Input: part model. Units: mm. Frame: model coordinates. A direction names the side the tool comes from. Give positions to 0.01 mm unless a question says otherwise; leave off trailing zeros. Write each loop counter-clockwise with the first axis right and the second up, starting at its lowest first coordinate (ties: lowest second). Pieces come first, ordered by that corner, then holes.
```python
from build123d import *

# Parameters (mm, degrees)
SKETCH21_R              = 5
CUT_EXTRUDE3_DEPTH      = 210.892061542
CUT_EXTRUDE3_DEPTH_BACK = 10.5


with BuildPart() as part:
    # Sweep-Thin3: sweep along a curve in space
    with BuildLine() as sweep_thin3_path:
        Line((0, 0, 0), (150, 0, 0))
        Line((150, 0, 0), (335.07515147, 200, 500))
        Line((335.07515147, 200, 500), (335.07515147, 200, 530))
    # Sketch2 → Sweep-Thin3 (sweep)
    with BuildSketch(Plane(origin=(0, 0, 0), x_dir=(0, 0, -1), z_dir=(1, 0, 0))):
        with BuildLine():
            Line((1.5, 9.5), (-1.5, 9.5))
            ThreePointArc((-1.5, 9.5), (-7.156854249, 7.156854249), (-9.5, 1.5))
            Line((-9.5, 1.5), (-9.5, -1.5))
            ThreePointArc((-9.5, -1.5), (-7.156854249, -7.156854249), (-1.5, -9.5))
            Line((-1.5, -9.5), (1.5, -9.5))
            ThreePointArc((1.5, -9.5), (7.156854249, -7.156854249), (9.5, -1.5))
            Line((9.5, -1.5), (9.5, 1.5))
            ThreePointArc((9.5, 1.5), (7.156854249, 7.156854249), (1.5, 9.5))
        make_face()
        with BuildLine():
            Line((1.5, 6.5), (-1.5, 6.5))
            ThreePointArc((-1.5, 6.5), (-5.035533906, 5.035533906), (-6.5, 1.5))
            Line((-6.5, 1.5), (-6.5, -1.5))
            ThreePointArc((-6.5, -1.5), (-5.035533906, -5.035533906), (-1.5, -6.5))
            Line((-1.5, -6.5), (1.5, -6.5))
            ThreePointArc((1.5, -6.5), (5.035533906, -5.035533906), (6.5, -1.5))
            Line((6.5, -1.5), (6.5, 1.5))
            ThreePointArc((6.5, 1.5), (5.035533906, 5.035533906), (1.5, 6.5))
        make_face(mode=Mode.SUBTRACT)
    sweep(path=sweep_thin3_path.line, transition=Transition.RIGHT)

    # Sketch21 → Cut-Extrude3 (cut, two sides)
    with BuildSketch(Plane(origin=(0, 0, 0), x_dir=(1, 0, 0), z_dir=(0, 1, 0))) as cut_extrude3_sk:
        with Locations((50, 0)):
            Circle(SKETCH21_R)
    extrude(amount=CUT_EXTRUDE3_DEPTH, mode=Mode.SUBTRACT)
    extrude(cut_extrude3_sk.sketch, amount=-CUT_EXTRUDE3_DEPTH_BACK, mode=Mode.SUBTRACT)


solid = part.part
```
Q1. Material intervals for line 1 along X through (y, z) = (-7, 0); line 2 along X through (y, z) = (-8.35, 0); line 3 along Z through (x, y) = (50, 7), sorted ascending.
Q2. Pin query (flat end, axial travel): pin 1 (0.9 mm diameter, centred on x = 26.5, z = -0.5, fed in from +Y); pin 2 (1.5 mm diameter, centred on x = 61.5, y = 0.5, fed in from +Z). Return the tip coordinate at first contact, or that it passes through.
Q3. Access query for faces 5 (the flat face through (251.49, 102.84, 247.66)), 6 (the flat face through (241.8, 107.6, 252.8)). Directions: +Z, -Z, +X, -X, +Y, -Y. A direction counts if a zero-diameter tool reaches every point of the face in a straight line with its end or side. Return the directions, or none.
Q4. Mould query, pull axis Z, two halves, no side actions, for faces 1 (the cylindrical face through (238.177, 105.393, 255.794)), 2 (the flat face through (328, 202, 530)), 3 (the cylindrical face through (251.78, 95.62, 250)), 4 (the flat face through (241.008, 110.553, 252.613)). Classes: +Z half, -Z half, draft (parallel to the pull), parting line (faces both ways), or undercut.
Q5. Section A-A, the plane x = 65. Return the cut outline in (y, z), then the cut area to 3 significant figures.
Solutions:
1. line 1: x = 0 to 45, 55 to 157.14
1. line 2: x = 0 to 45, 55 to 155.25
1. line 3: z = -7.31 to -5, 5 to 7.31
2. pin 1: stops at y = 9.5
2. pin 2: stops at z = 9.5
3. face 5: -Z, +X, +Y
3. face 6: none
4. face 1: undercut
4. face 2: +Z half
4. face 3: parting line
4. face 4: -Z half
5. outline: (-9.5, -1.5) arc R8 ccw to (-1.5, -9.5) - (1.5, -9.5) arc R8 ccw to (9.5, -1.5) - (9.5, 1.5) arc R8 ccw to (1.5, 9.5) - (-1.5, 9.5) arc R8 ccw to (-9.5, 1.5) - close; hole (-6.5, -1.5) arc R5 ccw to (-1.5, -6.5) - (1.5, -6.5) arc R5 ccw to (6.5, -1.5) - (6.5, 1.5) arc R5 ccw to (1.5, 6.5) - (-1.5, 6.5) arc R5 ccw to (-6.5, 1.5) - close
5. area: 159 mm2
